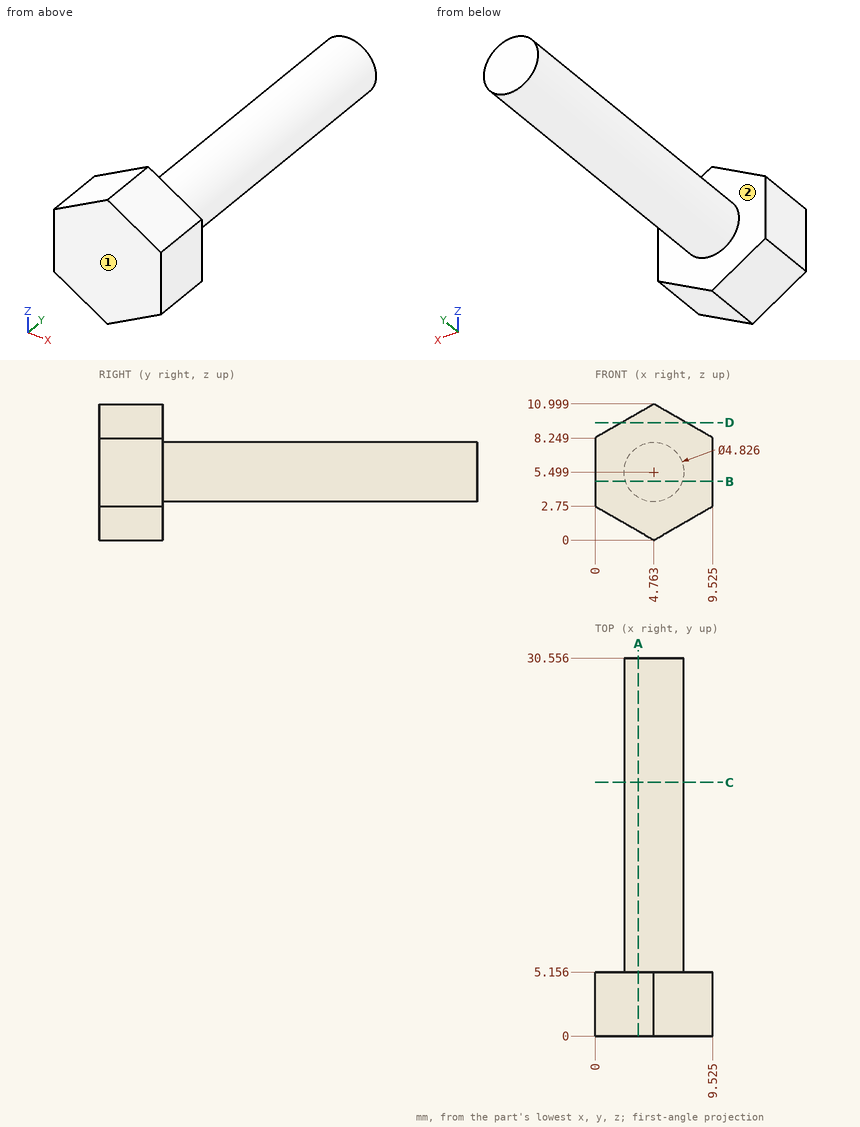
Verification items for this drawing (mm, ordinates from the low corner). A direction names the side the tool comes from. Round coordinates to 2 decimals unless told otherwise and drop trailing zeros. Order: outer loops, then holes, each group sorted by start corner. A loop starts at its lowest first (then second) coordinate and runs counter-clockwise, first axis right, second up. Notation, with made-up numbers: (82.5, -6.5) - (132.5, -6.5) arc R11 ccw to (132.5, 8.5) - close; hole circle Ø2 at (57.25, 3). An arc over 180 degrees is marked (long way). Use CSV: the item, a comma, the result in double quotes. Start each with the question number.
1) Section check D-D, the plane z = 9.5. Record the cut outline in (x, y).
2) Section check A-A, the plane x = 3.5. Record the cut outline in (y, z) (1 decimal), plus the area to 3 significant figures.
3) Thickness scan on L1, parallel to Y at x = 6.5, z = 1.5; L2, parallel to X at y = 21, z = 4 (1 decimal); L3, parallel to Z at x = 6.75, y = 24.5 (1 decimal). Record the ranges inside material, lowest first.
4) Go/stop test with flat-tipped pins: P1, Ø6, axis at y = 15, z = 4.5, coming from the +X side (1 decimal); P2, Ø1.5, axis at x = 3.5, y = 27, coming from the -Z side; P3, Ø5, axis at x = 5, y = 12.5, coming from the +Z side. Record where each tip stops, or that it passes through.
5) Section check C-C, the plane y = 20.5. Record the cut outline in (x, z) (1 decimal), plus the area to 3 significant figures.
6) Access from +Z, -Z, +X, -X, +Y, -Y to the whole of each face (thin tool, end or side, straight path). Record for the marked faces 1 and 2.
7) Section check B-B, the plane z = 4.75. Record the cut outline in (x, y) (1 decimal), plus the area to 3 significant figures.
Answers:
1,outline,"(2.17, 0) - (7.36, 0) - (7.36, 5.16) - (2.17, 5.16) - close"
2,outline,"(0, 0.7) - (5.2, 0.7) - (5.2, 3.4) - (30.6, 3.4) - (30.6, 7.6) - (5.2, 7.6) - (5.2, 10.3) - (0, 10.3) - close"
2,area,"154 mm²"
3,L1,"y = 0 to 5.16"
3,L2,"x = 2.9 to 6.7"
3,L3,"z = 4.1 to 6.9"
4,P1,"stops at x = 7.2"
4,P2,"stops at z = 3.14"
4,P3,"stops at z = 7.91"
5,outline,"circle Ø4.8 at (4.8, 5.5)"
5,area,"18.3 mm²"
6,face 1,"+Z, -Z, +X, -X, -Y"
6,face 2,"+Y"
7,outline,"(0, 0) - (9.5, 0) - (9.5, 5.2) - (7.1, 5.2) - (7.1, 30.6) - (2.5, 30.6) - (2.5, 5.2) - (0, 5.2) - close"
7,area,"166 mm²"
